Check sheet for the modelled part. Datum: model origin and axes. Units: mm. A direction names the side the tool comes from. Coordinates: 2 decimals unless noted, no trailing zeros. Loops run counter-clockwise (first coordinate to the right, second up) from the corner with the lowest first, then second, coordinate; pieces in that order, holes last. Notation, with made-up numbers: (12, 14) -> (49, 14) arc R32 cw to (49, 41) -> close; hole circle Ø5 at (36, -15.75). An arc over 180 degrees is marked (long way). Use CSV: the item, a comma, the result in double quotes.
```python
from build123d import *

# Parameters (mm, degrees)
SKETCH1_W                       = 26
SKETCH1_H                       = 26
BOSS_EXTRUDE1_DEPTH             = 2.5
BOSS_EXTRUDE2_REACH             = 20.554
BOSS_EXTRUDE2_DIRECTION_2_REACH = 20.554
BOSS_EXTRUDE3_DEPTH             = 20
BOSS_EXTRUDE3_DEPTH_BACK        = 20
FILLET1_R                       = 2
FILLET2_R                       = 1.5


with BuildPart() as part:
    # Sketch1 → Boss-Extrude1 (new body)
    with BuildSketch(Plane(origin=(0, 0, 0), x_dir=(1, 0, 0), z_dir=(0, 1, 0))):
        Rectangle(SKETCH1_W, SKETCH1_H)
    extrude(amount=BOSS_EXTRUDE1_DEPTH)

    # Boss-Extrude2: up to this face of the body (flat: up to its plane)
    boss_extrude2_end = Plane(part.part.faces().sort_by_distance((0, 1.25, 13))[0])
    # Sketch2 → Boss-Extrude2 (add, up to the picked face)
    with BuildSketch(Plane.XY, mode=Mode.PRIVATE) as boss_extrude2_sk1:
        with BuildLine():
            Line((10.529394514, -8), (10.529394514, 0))
            Line((10.529394514, 0), (0.170155306, 0))
            ThreePointArc((0.170155306, 0), (6.116867713, -2.319963995), (9.029394514, -8))
            Line((9.029394514, -8), (10.529394514, -8))
        make_face()
    boss_extrude2_tool1 = split(extrude(boss_extrude2_sk1.sketch, amount=BOSS_EXTRUDE2_REACH, mode=Mode.PRIVATE), bisect_by=boss_extrude2_end, keep=Keep.BOTH, mode=Mode.PRIVATE)
    # Sketch2 → Boss-Extrude2 (add, up to the picked face)
    with BuildSketch(Plane.XY, mode=Mode.PRIVATE) as boss_extrude2_sk2:
        with BuildLine():
            ThreePointArc((-8.859239207, -8), (-5.946712406, -2.319963995), (0, 0))
            Line((0, 0), (-10.359239207, 0))
            Line((-10.359239207, 0), (-10.359239207, -8))
            Line((-10.359239207, -8), (-8.859239207, -8))
        make_face()
    boss_extrude2_tool2 = split(extrude(boss_extrude2_sk2.sketch, amount=BOSS_EXTRUDE2_REACH, mode=Mode.PRIVATE), bisect_by=boss_extrude2_end, keep=Keep.BOTH, mode=Mode.PRIVATE)
    add(boss_extrude2_tool1.solids().sort_by(Axis((8.165693, -2.801403, 0), (0, 0, 1)))[0])
    add(boss_extrude2_tool2.solids().sort_by(Axis((-7.995538, -2.801403, 0), (0, 0, 1)))[0])

    # Boss-Extrude2 direction 2: up to this face of the body (flat: up to its plane)
    boss_extrude2_direction_2_end = Plane(part.part.faces().sort_by_distance((0, 1.25, -13))[0])
    # Sketch2 → Boss-Extrude2 direction 2 (add, up to the picked face)
    with BuildSketch(Plane.XY, mode=Mode.PRIVATE) as boss_extrude2_direction_2_sk1:
        with BuildLine():
            Line((10.529394514, -8), (10.529394514, 0))
            Line((10.529394514, 0), (0.170155306, 0))
            ThreePointArc((0.170155306, 0), (6.116867713, -2.319963995), (9.029394514, -8))
            Line((9.029394514, -8), (10.529394514, -8))
        make_face()
    boss_extrude2_direction_2_tool1 = split(extrude(boss_extrude2_direction_2_sk1.sketch, amount=-BOSS_EXTRUDE2_DIRECTION_2_REACH, mode=Mode.PRIVATE), bisect_by=boss_extrude2_direction_2_end, keep=Keep.BOTH, mode=Mode.PRIVATE)
    # Sketch2 → Boss-Extrude2 direction 2 (add, up to the picked face)
    with BuildSketch(Plane.XY, mode=Mode.PRIVATE) as boss_extrude2_direction_2_sk2:
        with BuildLine():
            ThreePointArc((-8.859239207, -8), (-5.946712406, -2.319963995), (0, 0))
            Line((0, 0), (-10.359239207, 0))
            Line((-10.359239207, 0), (-10.359239207, -8))
            Line((-10.359239207, -8), (-8.859239207, -8))
        make_face()
    boss_extrude2_direction_2_tool2 = split(extrude(boss_extrude2_direction_2_sk2.sketch, amount=-BOSS_EXTRUDE2_DIRECTION_2_REACH, mode=Mode.PRIVATE), bisect_by=boss_extrude2_direction_2_end, keep=Keep.BOTH, mode=Mode.PRIVATE)
    add(boss_extrude2_direction_2_tool1.solids().sort_by(Axis((8.165693, -2.801403, 0), (0, 0, -1)))[0])
    add(boss_extrude2_direction_2_tool2.solids().sort_by(Axis((-7.995538, -2.801403, 0), (0, 0, -1)))[0])

    # Sketch3 → Boss-Extrude3 (add, two sides: drawn at the far end of the back side and taken through both)
    with BuildSketch(Plane.XY.offset(-BOSS_EXTRUDE3_DEPTH_BACK)):
        with BuildLine():
            ThreePointArc((-8.859239207, -8), (-8.623127821, -6.726459638), (-8.206654057, -5.5))
            Line((-8.206654057, -5.5), (-9.58127784, -4.919828013))
            ThreePointArc((-9.58127784, -4.919828013), (-10.087515452, -6.430298336), (-10.359239207, -8))
            Line((-10.359239207, -8), (-8.859239207, -8))
        make_face()
        with BuildLine():
            Line((9.751433146, -4.919828013), (8.376809364, -5.5))
            ThreePointArc((8.376809364, -5.5), (8.793283128, -6.726459638), (9.029394514, -8))
            Line((9.029394514, -8), (10.529394514, -8))
            ThreePointArc((10.529394514, -8), (10.257670759, -6.430298336), (9.751433146, -4.919828013))
        make_face()
        with BuildLine():
            ThreePointArc((-2.5, -0.378845376), (-0.003485724, -3.3627e-05), (2.5, -0.329641118))
            Line((2.5, -0.329641118), (2.900351797, 1.107685747))
            ThreePointArc((2.900351797, 1.107685747), (-0.01816798, 1.491936382), (-2.928560564, 1.050324284))
            Line((-2.928560564, 1.050324284), (-2.5, -0.378845376))
        make_face()
    extrude(amount=BOSS_EXTRUDE3_DEPTH + BOSS_EXTRUDE3_DEPTH_BACK)

    # Fillet1
    fillet1_edges = [part.edges().sort_by_distance(p)[0] for p in [
        (13, 1.25, 13),
        (-13, 1.25, 13),
        (-13, 1.25, -13),
        (13, 1.25, -13),
    ]]
    fillet(fillet1_edges, radius=FILLET1_R)

    # Fillet2
    fillet2_edges = [part.edges().sort_by_distance(p)[0] for p in [
        (-10.359239207, 0, 0),
        (10.529394514, 0, 0),
    ]]
    fillet(fillet2_edges, radius=FILLET2_R)


solid = part.part
```
1) Cross-section at A-A on z = 14. Record the boundary of the cut face in (x, y).
Answer below:
outline,"(-10.36, -8) -> (-8.86, -8) arc R9 cw to (-8.21, -5.5) -> (-9.58, -4.92) arc R10.49 ccw to start; (-2.93, 1.05) -> (-2.5, -0.38) arc R9 cw to (2.5, -0.33) -> (2.9, 1.11) arc R10.49 ccw to start; (8.38, -5.5) arc R9 cw to (9.03, -8) -> (10.53, -8) arc R10.49 ccw to (9.75, -4.92) -> close"
2) Cross-section at B-B on y = -3. Record the boundary of the cut face in (x, z).
Answer below:
outline,"(-10.36, -13) -> (-6.62, -13) -> (-6.62, 13) -> (-10.36, 13) -> close; (6.79, -13) -> (10.53, -13) -> (10.53, 13) -> (6.79, 13) -> close"
3) Cross-section at C-C on z = 10. Record the boundary of the cut face in (x, y), and give its area (3 significant figures).
Answer below:
outline,"(-13, 0) -> (-11.86, 0) arc R1.5 cw to (-10.36, -1.5) -> (-10.36, -8) -> (-8.86, -8) arc R9 cw to (0, 0) -> (0.17, 0) arc R9 cw to (9.03, -8) -> (10.53, -8) -> (10.53, -1.5) arc R1.5 cw to (12.03, 0) -> (13, 0) -> (13, 2.5) -> (-13, 2.5) -> close"
area,"124 mm²"
4) Access from +Z, -Z, +X, -X, +Y, -Y to the whole of each face (thin tool, end or side, straight path). Record for faces 1 (the flat face through (-10.359, -5, 0)), 2 (the cylindrical face through (10.263, -6.452, -16.549)), 3 (the cylindrical face through (10.263, -6.452, 16.451)).
Answer below:
face 1,"+Z, -Z, -X, -Y"
face 2,"-Z, +X, +Y"
face 3,"+Z, +X, +Y"
5) Cross-section at D-D on x = 3.75. Record the boundary of the cut face in (y, z), and give its area (3 significant figures).
Answer below:
outline,"(-0.78, -13) -> (2.5, -13) -> (2.5, 13) -> (-0.78, 13) -> close"
area,"85.3 mm²"
6) Go/stop test with flat-tipped pins: pin 1 Ø2 at (y, z) = (-3.5, -1) entering from -X; pin 2 Ø3 at (x, y) = (-10, -5) entering from +Z; pin 3 Ø5 at (x, y) = (-9.5, 1) entering from +Z; pin 4 Ø0.8 at (x, z) = (12.5, -5) entering from -Y. Record where each tip stops, or that it passes through.
Answer below:
pin 1,"stops at x = -10.36"
pin 2,"stops at z = 20"
pin 3,"stops at z = 13"
pin 4,"stops at y = 0"
7) Draft check along Y on faces 4 (the cylindrical face through (-10.082, -6.409, 16.451)), 5 (the cylindrical face through (-12.4, 1.13, 12.43)), 6 (the flat face through (2.697, 0.379, 16.451)). Enter one of: released by +Y, released by -Y, zero draft, split by the parting line, or undercut.
Answer below:
face 4,"released by +Y"
face 5,"zero draft"
face 6,"released by -Y"
8) Thickness scan on line 1 along Z through (x, y) = (9.5, -2); line 2 along X through (y, z) = (-7.25, 18.5); line 3 along X through (y, z) = (-4.5, -1.5). Record the ranges inside material, lowest first. Write a range as from..to.
Answer below:
line 1,"z = -13..13"
line 2,"x = -10.26..-8.74, 8.91..10.43"
line 3,"x = -10.36..-7.71, 7.88..10.53"
